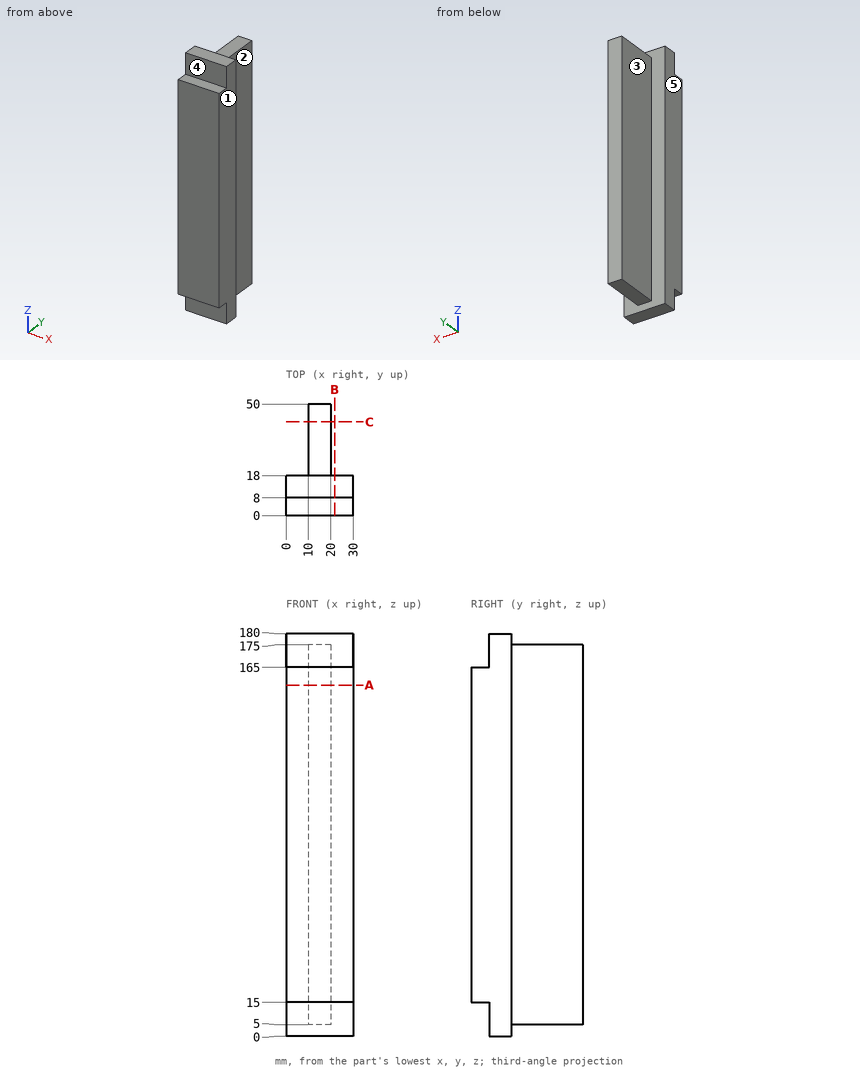
Source: three-view drawing plus pictorial views. Frame: mm from the lowest corner of the part. A direction names the side the tool comes from. Give positions to 0.01 mm unless a question says otherwise; leave off trailing zeros. Order: outer loops, then holes, each group sorted by start corner. A loop starts at its lowest first (then second) coordinate and runs counter-clockwise, first axis right, second up. Notation, with made-up numbers: M -21,36 L 25,36 A26 cw 25,52 Z; hole C -18.5,22.5 d4. An arc over 180 degrees is marked long. One line per question, with ' | ' between items. Start each with the question number.
1. Section query C-C (y = 42). Return the cut outline in (x, z), and give its area (3 significant figures).
2. Material intervals for probe 1 along Y at (x, z) = (24.5, 172); probe 2 along Y at (x, z) = (28, 40.5); probe 3 along Z at (x, y) = (15, 29.5), sorted ascending. Write a range as [from, to].
3. Section query B-B (x = 21.75). Return the cut outline in (y, z), and give its area (3 significant figures).
4. Section query A-A (z = 157). Return the cut outline in (x, y).
5. First-contact query: pin 1 Ø6 at (x, z) = (4, 85) entering from +Y; pin 2 Ø16 at (y, z) = (41.5, 56.5) entering from -X; pin 3 Ø12 at (x, y) = (17.5, 25.5) entering from +Z. Flat tips, straight axial feed; report the tip coordinate or a pass-through.
6. Access query for the marked faces 1, 2, 3, 4 and 5. Directions: +Z, -Z, +X, -X, +Y, -Y. A direction counts if a zero-diameter tool reaches every point of the face in a straight line with its end or side. Return the directions, or none.
Here are the results:
1) outline: M 10,5 L 20,5 L 20,175 L 10,175 Z | area: 1,700 mm²
2) probe 1: [8, 18] | probe 2: [0, 18] | probe 3: [5, 175]
3) outline: M 0,15 L 8,15 L 8,0 L 18,0 L 18,180 L 8,180 L 8,165 L 0,165 Z | area: 3,000 mm²
4) outline: M 0,0 L 30,0 L 30,18 L 20,18 L 20,50 L 10,50 L 10,18 L 0,18 Z
5) pin 1: y = 18 | pin 2: x = 10 | pin 3: z = 175
6) face 1: +Z, -Z, +X, +Y, -Y | face 2: +Z, -Z, +X, +Y | face 3: +Z, -Z, -X, +Y | face 4: +Z, +X, -X, -Y | face 5: +Z, -Z, -X, +Y, -Y
